Work out the finished part from the listing and answer in its coordinate system (mm). A direction names the side the tool comes from. Give positions to 0.01 mm unless a question says otherwise; leave off trailing zeros. Loops run counter-clockwise (first coordinate to the right, second up) from the corner with the lowest first, then second, coordinate; pieces in that order, holes last. Notation, with made-up numbers: M 78.25,47.25 L 103.25,47.25 A29 ccw 103.25,79.25 Z; hole C -11.5,48 d10. An arc over 180 degrees is marked long. Use a Markdown table: item, result.
```python
from build123d import *
from OCP.BRepAlgoAPI import BRepAlgoAPI_Cut
from OCP.TopTools import TopTools_ListOfShape

# Parameters (mm, degrees)
BOSS_EXTRUDE1_START = -12.501686
BOSS_EXTRUDE1_DEPTH = 25.003372
SKETCH4_R           = 7
CUT_EXTRUDE1_DEPTH  = 10


with BuildPart() as part:
    # Sketch2 → Loft1 section 0
    with BuildSketch(Plane.XY.offset(10)):
        with BuildLine():
            Line((-12.5, -12.5), (12.5, -12.5))
            Line((12.5, -12.5), (12.5, 12.5))
            Line((12.5, 12.5), (-12.5, 12.5))
            Line((-12.5, 12.5), (-12.5, -12.5))
        make_face()
    # Sketch1 for Loft1 → Loft1 section 1
    with BuildSketch(Plane.XY):
        with BuildLine():
            # circular arc as an exact rational Bezier (weights 1, cos(half-angle), 1)
            Bezier((-7.071067812, -7.071067812), (0, -14.142135623), (7.071067812, -7.071067812), weights=[1, 0.707106781, 1])
            Bezier((7.071067812, -7.071067812), (14.142135623, 0), (7.071067812, 7.071067812), weights=[1, 0.707106781, 1])
            Bezier((7.071067812, 7.071067812), (0, 14.142135623), (-7.071067812, 7.071067812), weights=[1, 0.707106781, 1])
            Bezier((-7.071067812, 7.071067812), (-14.142135623, 0), (-7.071067812, -7.071067812), weights=[1, 0.707106781, 1])
        make_face()
    loft()

    # Sketch3 → Boss-Extrude1 (add)
    with BuildSketch(Plane(origin=(0, 0, 0), x_dir=(0, 0, -1), z_dir=(1, 0, 0)).offset(BOSS_EXTRUDE1_START)):
        with BuildLine():
            Line((-10, 12.5), (-20, 12.5))
            ThreePointArc((-20, 12.5), (-32.5, 0), (-20, -12.5))
            Line((-20, -12.5), (-10, -12.5))
            Line((-10, -12.5), (-10, 12.5))
        make_face()
    extrude(amount=BOSS_EXTRUDE1_DEPTH)


with BuildPart() as cut_extrude1_tool:
    # Sketch4 → Cut-Extrude1 (new body)
    with BuildSketch(Plane(origin=(12.501685601, 0, 0), x_dir=(0, 0, -1), z_dir=(1, 0, 0))):
        with Locations((-20, 0)):
            Circle(SKETCH4_R)
    extrude(amount=-CUT_EXTRUDE1_DEPTH)


with BuildPart() as part_1:
    add(part.part)

    # Cut-Extrude1: cut by cut_extrude1_tool, with a tolerance
    cut_extrude1_stock = TopTools_ListOfShape()
    cut_extrude1_stock.Append(part_1.part.wrapped)
    cut_extrude1_tools = TopTools_ListOfShape()
    cut_extrude1_tools.Append(cut_extrude1_tool.part.wrapped)
    cut_extrude1_cut = BRepAlgoAPI_Cut()
    cut_extrude1_cut.SetArguments(cut_extrude1_stock)
    cut_extrude1_cut.SetTools(cut_extrude1_tools)
    cut_extrude1_cut.SetFuzzyValue(0.00001)
    cut_extrude1_cut.Build()
    add(Compound.cast(cut_extrude1_cut.Shape()).solids(), mode=Mode.REPLACE)


solid = part_1.part
```
(1) Given P1, Ø4, axis at y = 1, z = 17, coming from the +X side; P2, Ø1.5, axis at y = 5.5, z = 5, coming from the -X side; P3, Ø5, axis at y = -7, z = 4, coming from the -X side, each flat-ended and moving along its own axis, determine where each tip first touches the part or whether it passes through.
Entries:
| item | result |
|---|---|
| P1 | stops at x = 2.5 |
| P2 | stops at x = -11.08 |
| P3 | stops at x = -11.2 |
(2) A cutting plane is placed at A-A (z = 17). Write down the section's boundary in (x, y), and give its area (3 significant figures).
Entries:
| item | result |
|---|---|
| outline | M -12.5,-12.5 L 12.5,-12.5 L 12.5,-6.32 L 2.5,-6.32 L 2.5,6.32 L 12.5,6.32 L 12.5,12.5 L -12.5,12.5 Z |
| area | 499 mm² |
(3) Which of the six approach directions +Z, -Z, +X, -X, +Y, -Y give full straight-line access (tool end or side, diameter ignored) to faces 1 (the flat face through (2.502, 0, 20)), 2 (the flat face through (-12.502, 0, 21))?
Entries:
| item | result |
|---|---|
| face 1 | +X |
| face 2 | +Z, -Z, -X, +Y, -Y |
(4) The mould has two halves that part along Y. Classify faces 3 (the flat face through (12.502, 6, 26)), 4 (the cylindrical face through (-0.175, 0.275, 32.497)), 5 (the cylindrical face through (8, 0, 27)): released by +Y, released by -Y, zero draft, split by the parting line, or undercut.
Entries:
| item | result |
|---|---|
| face 3 | zero draft |
| face 4 | split by the parting line |
| face 5 | undercut |
(5) Consider probe 1 along Y at (x, z) = (8.25, 20); probe 2 along X at (y, z) = (2.25, 26.5); probe 3 along Z at (x, y) = (9.25, 1.75). Determine where each line is inside the solid, lowest interval first. Write a range as [from, to].
Entries:
| item | result |
|---|---|
| probe 1 | y = [-12.5, -7], [7, 12.5] |
| probe 2 | x = [-12.5, 2.5] |
| probe 3 | z = [0, 13.22], [26.78, 32.38] |
